Part model, mm, in its own coordinate system. Round coordinates to 2 decimals unless told otherwise and drop trailing zeros. Return JSON: item names as keys, results as strings. Group by question number.
(1) Drop a flat-ended pin along its axis: pin 1 Ø4 at (x, y) = (45.04, 529.97) entering from +Z. Give the stop position or say it passes through.
(2) Drill centre lines: L1, parallel to X at y = 74.5, z = 0.05; L2, parallel to X at y = 113, z = 0.05; L3, parallel to Y at x = 336.5, z = 0.05. Where is each one in solid material? Low to high. Write a range as from..to.
(3) Saw through at A-A (z = 0.05). State how many separate pieces and enclosed holes the cut face has, plus the area to 3 significant figures.
from build123d import *

# Parameters (mm, degrees)
BOSS_EXTRUDE1_DEPTH             = 0.127
BOSS_EXTRUDE2_DEPTH             = 0.127
F_1_4_0_25_DIAMETER_HOLE2_D     = 6.35
F_1_4_0_25_DIAMETER_HOLE3_D     = 6.35
F_1_4_0_25_DIAMETER_HOLE3_DEPTH = 0.127


with BuildPart() as part:
    # Sketch1 → Boss-Extrude1 (new body)
    with BuildSketch(Plane.XY):
        with BuildLine():
            Line((0, 0), (739.14, 0))
            add(Edge.make_bspline(
                [(277.420636668, 567.826315519), (496.859161811, 420.297110317), (620.758181585, 229.590161119), (739.14, 0)],
                knots=[0, 0, 0, 0, 1, 1, 1, 1], degree=3))
            Line((277.420636668, 567.826315519), (64.695636668, 567.826315519))
            Line((64.695636668, 567.826315519), (0, 0))
        make_face()
    extrude(amount=BOSS_EXTRUDE1_DEPTH)

    # Sketch5 → Boss-Extrude2 (add)
    with BuildSketch(Plane(origin=(0, 0, 0), x_dir=(-1, 0, 0), z_dir=(0, 0, -1))):
        Polygon((-64.695636668, 567.826315519), (-32.740222655, 567.826315519), (31.955414013, 0), (0, 0), align=None)
    extrude(amount=-BOSS_EXTRUDE2_DEPTH)

    # 1/4 (0.25) Diameter Hole2 (through all)
    with Locations(Plane.XY.offset(0.127)):
        with Locations((-6.712513837, 75.710175403), (-0.961790578, 126.183625671), (39.293272238, 479.49777755), (45.043995497, 529.971227818)):
            Hole(F_1_4_0_25_DIAMETER_HOLE2_D / 2)

    # 1/4 (0.25) Diameter Hole3
    with Locations(Plane.XY.offset(0.127)):
        with Locations((720.09, 12.7), (267.895636668, 555.126315519)):
            Hole(F_1_4_0_25_DIAMETER_HOLE3_D / 2, depth=F_1_4_0_25_DIAMETER_HOLE3_DEPTH)


solid = part.part
Computed values:
{
 "1": {"pin 1": "through"},
 "2": {"L1": "-23.47..-9.65, -3.78..699.67", "L2": "-19.08..678.24", "L3": "0..525.35"},
 "3": {"separate pieces": "1", "enclosed holes": "6", "area": "312,000 mm2"}
}
